Verification items for the finished model (mm, model axes). Give positions to 0.01 mm unless a question says otherwise; leave off trailing zeros. Loops run counter-clockwise (first coordinate to the right, second up) from the corner with the lowest first, then second, coordinate; pieces in that order, holes last. Notation, with made-up numbers: (5.5, -28) - (18.5, -28) arc R17 cw to (18.5, -20) - close; hole circle Ø6 at (18, 73.25). An arc over 180 degrees is marked (long way). Put each result on its own line as item: value. Start each with the question number.
```python
from build123d import *

# Parameters (mm, degrees)
SKETCH2_W           = 54.7846
SKETCH2_H           = 88.551
BOSS_EXTRUDE1_DEPTH = 3.175
SKETCH7_W           = 3.175
SKETCH7_H           = 18
SKETCH7_W_2         = 5
SKETCH7_H_2         = 3.175
SKETCH7_H_3         = 12.1
SKETCH7_W_3         = 14
CUT_EXTRUDE1_DEPTH  = 10
SKETCH8_W           = 62.7846
SKETCH8_H           = 96.551
SKETCH8_W_2         = 54.7846
SKETCH8_H_2         = 88.551
BOSS_EXTRUDE2_DEPTH = 3.175
SKETCH12_R          = 3.675
SKETCH12_R_2        = 1.675
BOSS_EXTRUDE4_DEPTH = 3.175
SKETCH13_R          = 1.675
CUT_EXTRUDE4_DEPTH  = 10
BOSS_EXTRUDE5_DEPTH = 3.175


with BuildPart() as part:
    # Sketch2 → Boss-Extrude1 (new body)
    with BuildSketch(Plane(origin=(0, 0, 0), x_dir=(1, 0, 0), z_dir=(0, 1, 0))):
        Rectangle(SKETCH2_W, SKETCH2_H)
    extrude(amount=BOSS_EXTRUDE1_DEPTH)

    # Sketch7 → Cut-Extrude1 (cut)
    with BuildSketch(Plane(origin=(0, 3.175, 0), x_dir=(1, 0, 0), z_dir=(0, 1, 0))):
        with Locations((-25.8048, 35.2755)):
            Rectangle(SKETCH7_W, SKETCH7_H)
        with Locations((-18.5173, 37.688)):
            Rectangle(SKETCH7_W_2, SKETCH7_H_2)
        with Locations((-11.2298, 38.2255)):
            Rectangle(SKETCH7_W, SKETCH7_H_3)
        Polygon((-6.4673, 44.2755), (-9.6423, 44.2755), (-9.6423, 32.1755), (-9.6423, 26.2755), (-6.4673, 26.2755), align=None)
        with Locations((8.875, 37.688)):
            Rectangle(SKETCH7_W_3, SKETCH7_H_2)
        with Locations((25.8048, 35.2755)):
            Rectangle(SKETCH7_W, SKETCH7_H)
        Polygon((24.2173, -10.3745), (24.2173, 7.6255), (24.2173, 20.6255), (21.0423, 20.6255), (21.0423, -10.3745), align=None)
        with Locations((25.8048, -1.3745)):
            Rectangle(SKETCH7_W, SKETCH7_H)
        with Locations((-8.0548, -1.3745)):
            Rectangle(SKETCH7_W, SKETCH7_H)
        with Locations((-25.8048, 0.0255)):
            Rectangle(SKETCH7_W, SKETCH7_H)
        with Locations((-25.8048, -35.2755)):
            Rectangle(SKETCH7_W, SKETCH7_H)
        with Locations((-8.0548, -35.2755)):
            Rectangle(SKETCH7_W, SKETCH7_H)
        with Locations((8.875, -37.688)):
            Rectangle(SKETCH7_W_3, SKETCH7_H_2)
        with Locations((25.8048, -35.2755)):
            Rectangle(SKETCH7_W, SKETCH7_H)
    extrude(amount=-CUT_EXTRUDE1_DEPTH, mode=Mode.SUBTRACT)

    # Sketch8 → Boss-Extrude2 (add)
    with BuildSketch(Plane(origin=(0, 3.175, 0), x_dir=(1, 0, 0), z_dir=(0, 1, 0))):
        Rectangle(SKETCH8_W, SKETCH8_H)
        Rectangle(SKETCH8_W_2, SKETCH8_H_2, mode=Mode.SUBTRACT)
    extrude(amount=-BOSS_EXTRUDE2_DEPTH)

    # Sketch12 → Boss-Extrude4 (add)
    # profile 1 of 4: a face of its own
    with BuildSketch(Plane(origin=(0, 3.175, 0), x_dir=(1, 0, 0), z_dir=(0, 1, 0))):
        with Locations((-31.3923, -48.2755)):
            Circle(SKETCH12_R)
        with Locations((-31.3923, -48.2755)):
            Circle(SKETCH12_R_2, mode=Mode.SUBTRACT)
    # profile 2 of 4: a face of its own
    with BuildSketch(Plane(origin=(0, 3.175, 0), x_dir=(1, 0, 0), z_dir=(0, 1, 0))):
        with Locations((31.3923, -48.2755)):
            Circle(SKETCH12_R)
        with Locations((31.3923, -48.2755)):
            Circle(SKETCH12_R_2, mode=Mode.SUBTRACT)
    # profile 3 of 4: a face of its own
    with BuildSketch(Plane(origin=(0, 3.175, 0), x_dir=(1, 0, 0), z_dir=(0, 1, 0))):
        with Locations((31.3923, 48.2755)):
            Circle(SKETCH12_R)
        with Locations((31.3923, 48.2755)):
            Circle(SKETCH12_R_2, mode=Mode.SUBTRACT)
    # profile 4 of 4: a face of its own
    with BuildSketch(Plane(origin=(0, 3.175, 0), x_dir=(1, 0, 0), z_dir=(0, 1, 0))):
        with Locations((-31.3923, 48.2755)):
            Circle(SKETCH12_R)
        with Locations((-31.3923, 48.2755)):
            Circle(SKETCH12_R_2, mode=Mode.SUBTRACT)
    extrude(amount=-BOSS_EXTRUDE4_DEPTH)

    # Sketch13 → Cut-Extrude4 (cut)
    with BuildSketch(Plane(origin=(0, 3.175, 0), x_dir=(1, 0, 0), z_dir=(0, 1, 0))):
        with Locations(Location((-31.3923, 48.2755, 0), (0, 0, 270))):
            Circle(SKETCH13_R)
        with Locations(Location((31.3923, 48.2755, 0), (0, 0, 270))):
            Circle(SKETCH13_R)
        with Locations(Location((31.3923, -48.2755, 0), (0, 0, 270))):
            Circle(SKETCH13_R)
        with Locations(Location((-31.3923, -48.2755, 0), (0, 0, 270))):
            Circle(SKETCH13_R)
    extrude(amount=-CUT_EXTRUDE4_DEPTH, mode=Mode.SUBTRACT)

    # Sketch14 → Boss-Extrude5 (add)
    with BuildSketch(Plane(origin=(0, 3.175, 0), x_dir=(1, 0, 0), z_dir=(0, 1, 0))):
        with BuildLine():
            Line((-35.0673, 48.2755), (-35.0673, -48.2755))
            ThreePointArc((-35.0673, -48.2755), (-33.990917421, -45.676882579), (-31.3923, -44.6005))
            Line((-31.3923, -44.6005), (-31.3923, 44.6005))
            ThreePointArc((-31.3923, 44.6005), (-33.990917421, 45.676882579), (-35.0673, 48.2755))
        make_face()
        with BuildLine():
            Line((31.392300042, 51.9505), (-31.3923, 51.9505))
            ThreePointArc((-31.3923, 51.9505), (-28.793682579, 50.874117421), (-27.7173, 48.2755))
            Line((-27.7173, 48.2755), (27.7173, 48.2755))
            ThreePointArc((27.7173, 48.2755), (28.793682594, 50.874117436), (31.392300042, 51.9505))
        make_face()
        with BuildLine():
            Line((-35.0673, 51.9505), (-35.0673, 48.2755))
            ThreePointArc((-35.0673, 48.2755), (-33.990917421, 50.874117421), (-31.3923, 51.9505))
            Line((-31.3923, 51.9505), (-35.0673, 51.9505))
        make_face()
        with BuildLine():
            ThreePointArc((31.3923, -44.6005), (33.990917421, -45.676882579), (35.0673, -48.2755))
            Line((35.0673, -48.2755), (35.0673, 48.2755))
            ThreePointArc((35.0673, 48.2755), (33.990917421, 45.676882579), (31.3923, 44.6005))
            Line((31.3923, 44.6005), (31.3923, -44.6005))
        make_face()
        with BuildLine():
            ThreePointArc((31.392300042, 51.9505), (33.990917436, 50.874117406), (35.0673, 48.2755))
            Line((35.0673, 48.2755), (35.0673, 51.9505))
            Line((35.0673, 51.9505), (31.392300042, 51.9505))
        make_face()
        with BuildLine():
            ThreePointArc((35.0673, -48.2755), (33.990917421, -50.874117421), (31.3923, -51.9505))
            Line((31.3923, -51.9505), (35.0673, -51.9505))
            Line((35.0673, -51.9505), (35.0673, -48.2755))
        make_face()
        with BuildLine():
            ThreePointArc((-27.7173, -48.2755), (-28.793682579, -50.874117421), (-31.3923, -51.9505))
            Line((-31.3923, -51.9505), (31.3923, -51.9505))
            ThreePointArc((31.3923, -51.9505), (28.793682579, -50.874117421), (27.7173, -48.2755))
            Line((27.7173, -48.2755), (-27.7173, -48.2755))
        make_face()
        with BuildLine():
            Line((-35.0673, -48.2755), (-35.0673, -51.9505))
            Line((-35.0673, -51.9505), (-31.3923, -51.9505))
            ThreePointArc((-31.3923, -51.9505), (-33.990917421, -50.874117421), (-35.0673, -48.2755))
        make_face()
    extrude(amount=-BOSS_EXTRUDE5_DEPTH)


solid = part.part
```
1) Section check A-A, the plane x = -8. Enter the section's corners in (y, z) (1 decimal).
2) Section check C-C, the plane x = 23. Enter the section's corners in (y, z) (1 decimal), plus the area to 3 significant figures.
3) Section check B-B, the plane z = -35. Enter the section's corners in (x, y) (3 decimals), plus the area to 3 significant figures.
4) Scan lines: line 1 along X through (y, z) = (2.6, -2); line 2 along X through (y, z) = (0.4, 34.5); line 3 along X through (y, z) = (0.2, -39) (3 decimals). Record each from-to range of solid material in increasing order. Write a range as from..to.
5) Depth check by flat-ended pin: P1, Ø2, axis at x = 31.39, z = -48.28, coming from the -Y side. Enter the tip coordinate at first touch or a pass-through.
6) Section check D-D, the plane y = 2. State how many separate pieces and enclosed holes the cut face has, plus the area to 3 significant figures.
7) Draft check along Z on faces 1 (the face through (-35.067, 2, -1)), 2 (the face through (-26, 2, 8.974)). Enter one of: pulls with the +Z half, pulls with the -Z half, needs draft (parallel to the pull), parting line crosses it, or undercut.
Results are:
1. outline: (0, -52) - (3.2, -52) - (3.2, -44.3) - (0, -44.3) - close; (0, -26.3) - (3.2, -26.3) - (3.2, -7.6) - (0, -7.6) - close; (0, 10.4) - (3.2, 10.4) - (3.2, 26.3) - (0, 26.3) - close; (0, 44.3) - (3.2, 44.3) - (3.2, 52) - (0, 52) - close
2. outline: (0, -52) - (3.2, -52) - (3.2, -20.6) - (0, -20.6) - close; (0, 10.4) - (3.2, 10.4) - (3.2, 52) - (0, 52) - close
2. area: 231 mm2
3. outline: (-35.067, 0) - (-27.392, 0) - (-27.392, 3.175) - (-35.067, 3.175) - close; (-24.217, 0) - (-12.817, 0) - (-12.817, 3.175) - (-24.217, 3.175) - close; (-6.467, 0) - (24.217, 0) - (24.217, 3.175) - (-6.467, 3.175) - close; (27.392, 0) - (35.067, 0) - (35.067, 3.175) - (27.392, 3.175) - close
3. area: 182 mm2
4. line 1: x = -35.07..-27.39, -24.22..-9.64, -6.47..21.04, 27.39..35.07
4. line 2: x = -35.07..-27.39, -24.22..-9.64, -6.47..24.22, 27.39..35.07
4. line 3: x = -35.067..-27.392, -24.217..-21.017, -16.017..-12.817, -6.467..1.875, 15.875..24.217, 27.392..35.067
5. P1: passes through
6. separate pieces: 1
6. enclosed holes: 16
6. area: 6,500 mm2
7. face 1: needs draft
7. face 2: undercut
